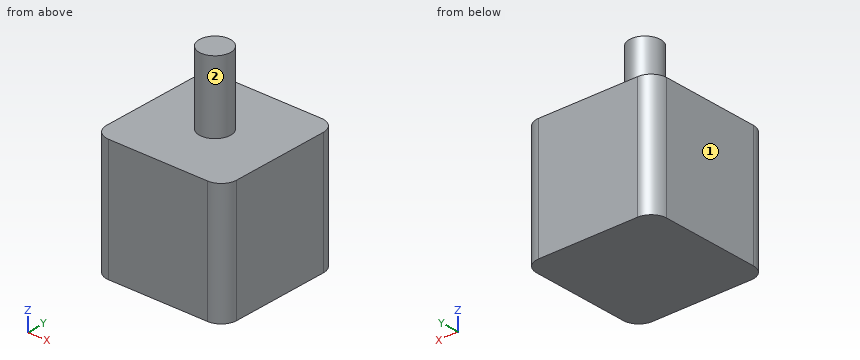
from build123d import *

# Parameters (mm, degrees)
ESQUISSE1_W             = 42
ESQUISSE1_H             = 42
BOSS_EXTRU_1_DEPTH      = 39
CONG_1_R                = 5
ESQUISSE2_R             = 5
BOSS_EXTRU_2_DEPTH      = 23
ESQUISSE3_R             = 5
BOSS_EXTRU_3_DEPTH      = 85
ESQUISSE4_R             = 5
ENL_V_MAT_EXTRU_1_DEPTH = 23


with BuildPart() as part:
    # Esquisse1 → Boss.-Extru.1 (new body)
    with BuildSketch(Plane.XY):
        with Locations((21, -21)):
            Rectangle(ESQUISSE1_W, ESQUISSE1_H)
    extrude(amount=BOSS_EXTRU_1_DEPTH)

    # Congé1
    cong_1_edges = [part.edges().sort_by_distance(p)[0] for p in [
        (0, 0, 19.5),
        (42, 0, 19.5),
        (42, -42, 19.5),
        (0, -42, 19.5),
    ]]
    fillet(cong_1_edges, radius=CONG_1_R)

    # Esquisse2 → Boss.-Extru.2 (add)
    with BuildSketch(Plane(origin=(0, 0, 0), x_dir=(-1, 0, 0), z_dir=(0, 0, -1))):
        with Locations((-21, -21)):
            Circle(ESQUISSE2_R)
    extrude(amount=BOSS_EXTRU_2_DEPTH)

    # Esquisse3 → Boss.-Extru.3 (add)
    with BuildSketch(Plane(origin=(0, 0, -23), x_dir=(-1, 0, 0), z_dir=(0, 0, -1))):
        with Locations((-21, -21)):
            Circle(ESQUISSE3_R)
    extrude(amount=-BOSS_EXTRU_3_DEPTH)

    # Esquisse4 → Enlèv. mat.-Extru.1 (cut)
    with BuildSketch(Plane(origin=(0, 0, -23), x_dir=(-1, 0, 0), z_dir=(0, 0, -1))):
        with Locations((-21, -21)):
            Circle(ESQUISSE4_R)
    extrude(amount=-ENL_V_MAT_EXTRU_1_DEPTH, mode=Mode.SUBTRACT)


solid = part.part
The model under review builds one solid part; all positions refer to its coordinate system, in mm. Face numbers are marked on the shaded views. A direction names the side the tool comes from. Round coordinates to 2 decimals unless told otherwise and drop trailing zeros. Order: outer loops, then holes, each group sorted by start corner. A loop starts at its lowest first (then second) coordinate and runs counter-clockwise, first axis right, second up. Notation, with made-up numbers: (89.5, -33.5) -> (138.5, -33.5) arc R14 ccw to (138.5, -11.5) -> close; hole circle Ø11 at (-36, 44). An arc over 180 degrees is marked (long way). Return JSON: item names as keys, results as strings.
1. For the marked faces 1 and 2, list the 3-axis set-ups (+Z, -Z, +X, -X, +Y, -Y) from which the entire face can be reached by the end or side of a thin tool; tool diameter is ignored.
Answer block:
{"face 1": "+Z, -Z, -X, +Y, -Y", "face 2": "+Z"}
2. Take a section at C-C (z = 40). Write out the cut boundary in (x, y), then the cut area to 3 significant figures.
Answer block:
{"outline": "circle Ø10 at (21, -21)", "area": "78.5 mm²"}
3. For L1, parallel to Z at x = 39.5, y = -10.5; L2, parallel to Y at x = 21, z = 43; L3, parallel to X at y = -3.5, z = 12.5, list the stretches that pass through material, from the lowest coordinate up. Write a range as [from, to].
Answer block:
{"L1": "z = [0, 39]", "L2": "y = [-26, -16]", "L3": "x = [0.23, 41.77]"}
4. Take a section at A-A (y = -21). Write out the cut boundary in (x, z), then the cut area to 3 significant figures.
Answer block:
{"outline": "(0, 0) -> (42, 0) -> (42, 39) -> (26, 39) -> (26, 62) -> (16, 62) -> (16, 39) -> (0, 39) -> close", "area": "1,870 mm²"}
5. Take a section at D-D (x = 27.5). Write out the cut boundary in (y, z), then the cut area to 3 significant figures.
Answer block:
{"outline": "(-42, 0) -> (0, 0) -> (0, 39) -> (-42, 39) -> close", "area": "1,640 mm²"}
6. Take a section at B-B (x = 21). Write out the cut boundary in (y, z).
Answer block:
{"outline": "(-42, 0) -> (0, 0) -> (0, 39) -> (-16, 39) -> (-16, 62) -> (-26, 62) -> (-26, 39) -> (-42, 39) -> close"}
